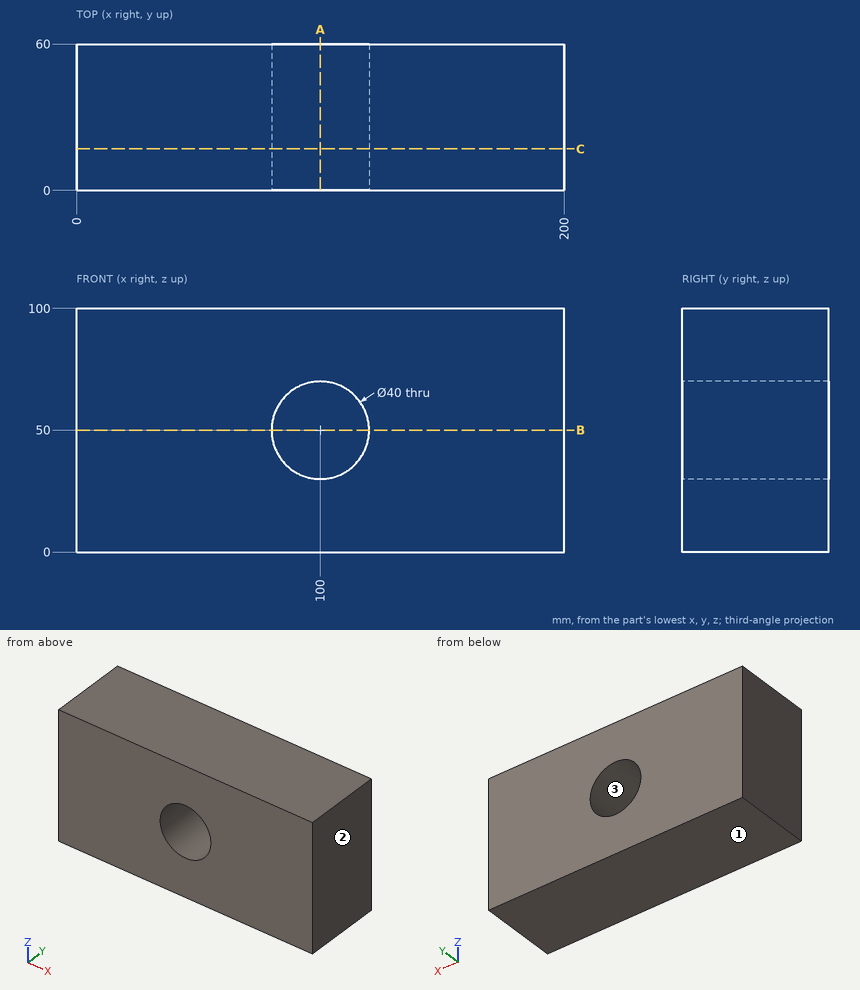
Could you check a few things on this drawing? It's one solid part, dimensions in mm from its lowest x, y, z. Give positions to 0.01 mm unless a question says otherwise; leave off trailing zeros. Loops run counter-clockwise (first coordinate to the right, second up) from the corner with the lowest first, then second, coordinate; pieces in that order, holes last. Notation, with made-up numbers: (80, 89) -> (93, 89) arc R15 ccw to (93, 107) -> close; hole circle Ø8 at (-6, 10.25). An arc over 180 degrees is marked (long way). Use one line per item in the form item = value. Start each with the question number.
1) Imagine slicing it at A-A (x = 100). Please give me the cut outline in (y, z), then the cut area to 3 significant figures.
2) Please list where these lines run through material, in increasing order: line 1 along Z through (x, y) = (100, 27); line 2 along Z through (x, y) = (82, 45); line 3 along X through (y, z) = (55, 32.5).
3) Imagine slicing it at C-C (y = 17). Please give me the cut outline in (x, z), then the cut area to 3 significant figures.
4) Thinking about a two-plate mould opening in Z: for the marked faces 1, 2 and 3, which applies, +Z half, -Z half, draft (parallel to the pull), parting line (faces both ways), or undercut?
5) Imagine slicing it at B-B (z = 50). Please give me the cut outline in (x, y), then the cut area to 3 significant figures.
6) For P1, Ø8, axis at x = 97.5, z = 82, coming from the -Y side; P2, Ø4, axis at x = 103, z = 33, coming from the -Y side, each with a flat end and sliding along its axis, tell me the tip position at first contact or that it passes through.
Check values:
q1.outline = (0, 0) -> (60, 0) -> (60, 30) -> (0, 30) -> close; (0, 70) -> (60, 70) -> (60, 100) -> (0, 100) -> close
q1.area = 3,600 mm^2
q2.line_1 = 0 to 30, 70 to 100
q2.line_2 = 0 to 41.28, 58.72 to 100
q2.line_3 = 0 to 90.32, 109.68 to 200
q3.outline = (0, 0) -> (200, 0) -> (200, 100) -> (0, 100) -> close; hole circle Ø40 at (100, 50)
q3.area = 18,700 mm^2
q4.face_1 = -Z half
q4.face_2 = draft
q4.face_3 = undercut
q5.outline = (0, 0) -> (80, 0) -> (80, 60) -> (0, 60) -> close; (120, 0) -> (200, 0) -> (200, 60) -> (120, 60) -> close
q5.area = 9,600 mm^2
q6.P1 = 0
q6.P2 = through
